Check sheet for the modelled part. Datum: model origin and axes. Units: mm. Coordinates: 2 decimals unless noted, no trailing zeros. Loops run counter-clockwise (first coordinate to the right, second up) from the corner with the lowest first, then second, coordinate; pieces in that order, holes last. Notation, with made-up numbers: (45, 13) -> (73, 13) arc R28 ccw to (73, 32) -> close; hole circle Ø7 at (88, 65). An arc over 180 degrees is marked (long way). Use one line per item in the form item = value.
from build123d import *

# Parameters (mm, degrees)
BOSS_EXTRUDE1_DEPTH = 2.5


with BuildPart() as part:
    # Sketch2 → Boss-Extrude1 (new, symmetric)
    with BuildSketch(Plane.XY):
        Polygon((-1336.454343847, -212.29700175), (-1336.454343847, -207.29700175), (-1321.70434708, -207.29700175), (-1321.70434708, -197.04700175), (-1316.20434708, -197.04700175), (-1316.20434708, -207.29700175), (-1306.70434708, -207.29700175), (-1306.70434708, -197.04700175), (-1301.20434708, -197.04700175), (-1301.20434708, -207.29700175), (-1286.454340614, -207.29700175), (-1286.454340614, -212.29700175), (-1276.454340614, -212.29700175), (-1276.454340614, -182.29700175), (-1286.454340614, -182.29700175), (-1286.454340614, -187.29700175), (-1336.454343847, -187.29700175), (-1336.454343847, -182.29700175), (-1356.454343847, -182.29700175), (-1356.454343847, -187.29700175), (-1406.454340614, -187.29700175), (-1406.454340614, -182.29700175), (-1416.454340614, -182.29700175), (-1416.454340614, -212.29700175), (-1406.454340614, -212.29700175), (-1406.454340614, -207.29700175), (-1391.704340614, -207.29700175), (-1391.704340614, -197.04700175), (-1386.204340614, -197.04700175), (-1386.204340614, -207.29700175), (-1376.704340614, -207.29700175), (-1376.704340614, -197.04700175), (-1371.204340614, -197.04700175), (-1371.204340614, -207.29700175), (-1356.454343847, -207.29700175), (-1356.454343847, -212.29700175), align=None)
    extrude(amount=BOSS_EXTRUDE1_DEPTH, both=True)


solid = part.part
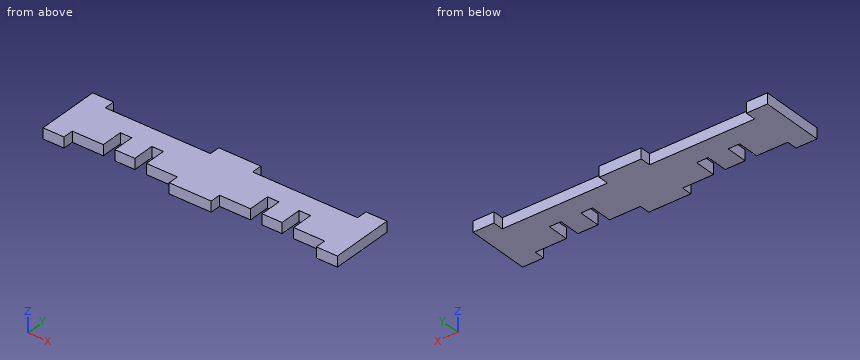
(1) Section check C-C, the plane x = -1398.5. Record the boundary of the cut face in (y, z).
Established:
outline = (-207.3, -2.5) -> (-187.3, -2.5) -> (-187.3, 2.5) -> (-207.3, 2.5) -> close
(2) Section check A-A, the plane y = -186. Record the boundary of the cut face in (x, z).
Established:
outline = (-1416.45, -2.5) -> (-1406.45, -2.5) -> (-1406.45, 2.5) -> (-1416.45, 2.5) -> close; (-1356.45, -2.5) -> (-1336.45, -2.5) -> (-1336.45, 2.5) -> (-1356.45, 2.5) -> close; (-1286.45, -2.5) -> (-1276.45, -2.5) -> (-1276.45, 2.5) -> (-1286.45, 2.5) -> close
(3) Scan lines: line 1 along X through (y, z) = (-202.5, 1.5); line 2 along X through (y, z) = (-209.5, 0.4); line 3 along Y through (x, z) = (-1405, 2.25). Record each from-to range of solid material in increasing order.
Established:
line_1 = -1416.45 to -1391.7, -1386.2 to -1376.7, -1371.2 to -1321.7, -1316.2 to -1306.7, -1301.2 to -1276.45
line_2 = -1416.45 to -1406.45, -1356.45 to -1336.45, -1286.45 to -1276.45
line_3 = -207.3 to -187.3
(4) Go/stop test with a flat-tipped pin: P1, Ø1.5, axis at x = -1389, z = -1, coming from the -Y side. Record where the tip stops, or that it passes through.
Established:
P1 = -197.05
(5) Section check B-B, the plane y = -206. Record the boundary of the cut face in (x, z), plus the area to 3 significant figures.
Established:
outline = (-1416.45, -2.5) -> (-1391.7, -2.5) -> (-1391.7, 2.5) -> (-1416.45, 2.5) -> close; (-1386.2, -2.5) -> (-1376.7, -2.5) -> (-1376.7, 2.5) -> (-1386.2, 2.5) -> close; (-1371.2, -2.5) -> (-1321.7, -2.5) -> (-1321.7, 2.5) -> (-1371.2, 2.5) -> close; (-1316.2, -2.5) -> (-1306.7, -2.5) -> (-1306.7, 2.5) -> (-1316.2, 2.5) -> close; (-1301.2, -2.5) -> (-1276.45, -2.5) -> (-1276.45, 2.5) -> (-1301.2, 2.5) -> close
area = 590 mm²
